Here's how the part is built. I have some questions about the finished solid (model axes, mm). Round coordinates to 2 decimals unless told otherwise and drop trailing zeros. One line per item, written item: value.
from build123d import *

# Parameters (mm, degrees)
SKETCH1_W                          = 410
SKETCH1_H                          = 360
BOSS_EXTRUDE1_DEPTH                = 18
SKETCH2_R                          = 12.5
CAMERA_STAND_TO_BASE_PROFILE_DEPTH = 546.915744415
SKETCH3_R                          = 2
CUT_EXTRUDE2_DEPTH                 = 546.915744415
SKETCH6_R                          = 2
CAMERA_STAND_TO_BASE_SCREW_DEPTH   = 546.915744415
SKETCH7_R                          = 4
CUT_EXTRUDE3_DEPTH                 = 8


with BuildPart() as part:
    # Sketch1 → Boss-Extrude1 (new body)
    with BuildSketch(Plane(origin=(0, 0, 0), x_dir=(1, 0, 0), z_dir=(0, 1, 0))):
        with Locations((205, 180)):
            Rectangle(SKETCH1_W, SKETCH1_H)
    extrude(amount=BOSS_EXTRUDE1_DEPTH)

    # Sketch2 → Camera Stand to Base (Profile) (cut, through all)
    with BuildSketch(Plane(origin=(0, 18, 0), x_dir=(1, 0, 0), z_dir=(0, 1, 0))):
        with Locations(Location((205, 335, 0), (0, 0, 270))):
            Circle(SKETCH2_R)
    extrude(amount=-CAMERA_STAND_TO_BASE_PROFILE_DEPTH, mode=Mode.SUBTRACT)

    # Sketch3 → Cut-Extrude2 (cut, through all)
    with BuildSketch(Plane(origin=(0, 18, 0), x_dir=(1, 0, 0), z_dir=(0, 1, 0))):
        with Locations(Location((40, 40, 0), (0, 0, 270))):
            Circle(SKETCH3_R)
        with Locations(Location((50, 40, 0), (0, 0, 270))):
            Circle(SKETCH3_R)
        with Locations(Location((360, 40, 0), (0, 0, 270))):
            Circle(SKETCH3_R)
        with Locations(Location((370, 40, 0), (0, 0, 270))):
            Circle(SKETCH3_R)
        with Locations(Location((370, 270, 0), (0, 0, 270))):
            Circle(SKETCH3_R)
        with Locations(Location((360, 270, 0), (0, 0, 270))):
            Circle(SKETCH3_R)
        with Locations(Location((40, 270, 0), (0, 0, 270))):
            Circle(SKETCH3_R)
        with Locations(Location((50, 270, 0), (0, 0, 270))):
            Circle(SKETCH3_R)
    extrude(amount=-CUT_EXTRUDE2_DEPTH, mode=Mode.SUBTRACT)

    # Sketch6 → Camera Stand to Base (Screw) (cut, through all)
    with BuildSketch(Plane.XZ):
        with Locations(Location((205, -308, 0), (0, 0, 270))):
            Circle(SKETCH6_R)
        with Locations(Location((178, -335, 0), (0, 0, 270))):
            Circle(SKETCH6_R)
        with Locations(Location((232, -335, 0), (0, 0, 270))):
            Circle(SKETCH6_R)
    extrude(amount=-CAMERA_STAND_TO_BASE_SCREW_DEPTH, mode=Mode.SUBTRACT)

    # Sketch7 → Cut-Extrude3 (cut)
    with BuildSketch(Plane.XZ):
        with Locations(Location((40, -40, 0), (0, 0, 270))):
            Circle(SKETCH7_R)
        with Locations(Location((50, -40, 0), (0, 0, 270))):
            Circle(SKETCH7_R)
        with Locations(Location((360, -40, 0), (0, 0, 270))):
            Circle(SKETCH7_R)
        with Locations(Location((370, -40, 0), (0, 0, 270))):
            Circle(SKETCH7_R)
        with Locations(Location((370, -270, 0), (0, 0, 270))):
            Circle(SKETCH7_R)
        with Locations(Location((360, -270, 0), (0, 0, 270))):
            Circle(SKETCH7_R)
        with Locations(Location((50, -270, 0), (0, 0, 270))):
            Circle(SKETCH7_R)
        with Locations(Location((40, -270, 0), (0, 0, 270))):
            Circle(SKETCH7_R)
        with Locations(Location((178, -335, 0), (0, 0, 270))):
            Circle(SKETCH7_R)
        with Locations(Location((205, -308, 0), (0, 0, 270))):
            Circle(SKETCH7_R)
        with Locations(Location((232, -335, 0), (0, 0, 270))):
            Circle(SKETCH7_R)
    extrude(amount=-CUT_EXTRUDE3_DEPTH, mode=Mode.SUBTRACT)


solid = part.part
Q1. If I drill on line 1 along X through (y, z) = (15.5, -270); line 2 along Z through (x, y) = (360, 2); line 3 along X through (y, z) = (6, -40), over which ranges is the centre line in solid material (lowest first)?
Results list:
line 1: 0 to 38, 42 to 48, 52 to 358, 362 to 368, 372 to 410
line 2: -360 to -274, -266 to -44, -36 to 0
line 3: 0 to 36, 44 to 46, 54 to 356, 364 to 366, 374 to 410
Q2. Will these pins go through, and if not, where does the flat tip stop? pin 1 (6 mm diameter, centred on x = 298, z = -304.5, fed in from -Y); pin 2 (4.5 mm diameter, centred on x = 40, z = -270, fed in from -Y).
Results list:
pin 1: y = 0
pin 2: y = 8
Q3. We'd pull the mould along Z, two halves only. Please class faces 1 (the cylindrical face through (215.54, 9.13, -328.28)), 2 (the flat face through (202, 9, -360)), 3 (the flat face through (0, 9, -177)): released by +Z, released by -Z, zero draft, split by the parting line, or undercut.
Results list:
face 1: undercut
face 2: released by -Z
face 3: zero draft
